```python
from build123d import *

# Parameters (mm, degrees)
SKETCH1_W           = 110
SKETCH1_H           = 50
SKETCH1_R           = 17.5
BOSS_EXTRUDE1_DEPTH = 6
SKETCH2_W           = 110
SKETCH2_H           = 7
BOSS_EXTRUDE2_DEPTH = 65
BOSS_EXTRUDE3_DEPTH = 6
BOSS_EXTRUDE4_DEPTH = 6
CUT_EXTRUDE1_REACH  = 52
SKETCH5_R           = 15
SKETCH6_R           = 3
CUT_EXTRUDE2_DEPTH  = 7
SKETCH7_R           = 2
CUT_EXTRUDE3_DEPTH  = 51


with BuildPart() as part:
    # Sketch1 → Boss-Extrude1 (new body)
    with BuildSketch(Plane(origin=(0, 0, 0), x_dir=(1, 0, 0), z_dir=(0, 1, 0))):
        Rectangle(SKETCH1_W, SKETCH1_H)
        Circle(SKETCH1_R, mode=Mode.SUBTRACT)
    extrude(amount=BOSS_EXTRUDE1_DEPTH)

    # Sketch2 → Boss-Extrude2 (add)
    with BuildSketch(Plane(origin=(0, 6, 0), x_dir=(1, 0, 0), z_dir=(0, 1, 0))):
        with Locations((0, -21.5)):
            Rectangle(SKETCH2_W, SKETCH2_H)
    extrude(amount=BOSS_EXTRUDE2_DEPTH)

    # Sketch3 → Boss-Extrude3 (add)
    with BuildSketch(Plane(origin=(55, 0, 0), x_dir=(0, 0, -1), z_dir=(1, 0, 0))):
        Polygon((-18, 6), (25, 6), (-18, 49), align=None)
    extrude(amount=-BOSS_EXTRUDE3_DEPTH)

    # Sketch4 → Boss-Extrude4 (add)
    with BuildSketch(Plane.ZY.offset(55)):
        Polygon((-25, 6), (18, 6), (18, 49), align=None)
    extrude(amount=-BOSS_EXTRUDE4_DEPTH)

    # Sketch5 → Cut-Extrude1 (cut, up to next)
    with BuildSketch(Plane.XY.offset(25), mode=Mode.PRIVATE) as cut_extrude1_sk1:
        with Locations((0, 46)):
            Circle(SKETCH5_R)
    cut_extrude1_tool1 = extrude(cut_extrude1_sk1.sketch, amount=-CUT_EXTRUDE1_REACH, mode=Mode.PRIVATE) & part.part
    add(cut_extrude1_tool1.solids().sort_by_distance((0, 46, 25))[0], mode=Mode.SUBTRACT)

    # Sketch6 → Cut-Extrude2 (cut, through all)
    with BuildSketch(Plane(origin=(0, 6, 0), x_dir=(1, 0, 0), z_dir=(0, 1, 0))):
        with Locations((-41.329699244, 20)):
            Circle(SKETCH6_R)
        with Locations((-41.329699244, -13)):
            Circle(SKETCH6_R)
        with Locations((41.329699244, -13)):
            Circle(SKETCH6_R)
        with Locations((41.329699244, 20)):
            Circle(SKETCH6_R)
    extrude(amount=-CUT_EXTRUDE2_DEPTH, mode=Mode.SUBTRACT)

    # Sketch7 → Cut-Extrude3 (cut, through all)
    with BuildSketch(Plane.XY.offset(25)):
        with Locations((-27, 65)):
            Circle(SKETCH7_R)
        with Locations((27, 65)):
            Circle(SKETCH7_R)
        with Locations((-27, 11)):
            Circle(SKETCH7_R)
        with Locations((27, 11)):
            Circle(SKETCH7_R)
    extrude(amount=-CUT_EXTRUDE3_DEPTH, mode=Mode.SUBTRACT)


solid = part.part
```
Read the model definition and answer for the solid it produces. Units are mm, in the model's axes. A direction names the side the tool comes from. Coordinates: 2 decimals unless noted, no trailing zeros. Order: outer loops, then holes, each group sorted by start corner. A loop starts at its lowest first (then second) coordinate and runs counter-clockwise, first axis right, second up. Notation, with made-up numbers: (26, 76.25) - (64, 76.25) arc R19 cw to (64, 88.25) - close; hole circle Ø8 at (10, 13). An arc over 180 degrees is marked (long way). Answer as a JSON object with one key per item and string values. Group by question number.
Item 1: The mould has two halves that part along Y. Classify faces 1 (the face through (-13, 0, 16)), 2 (the face through (-25.092, 11.601, 21.549)), 3 (the face through (-49, 18, 6)): +Y half, -Y half, draft (parallel to the pull), parting line (faces both ways), or undercut.
Item 2: Section B-B (y = 46) is taken. Give the vertices of the cut face in (x, z).
Item 3: A tool of negligible diameter and unlimited length cuts with its end or side. For faces 4 (the face through (-13.887, 2.958, 10.648)), 5 (the face through (-0.8, 30.8, 18)), from which of +Z, -Z, +X, -X, +Y, -Y can it reach the whole face along a straight path? Write none if from no direction.
Item 4: Section A-A (x = -27) is taken. Give the vertices of the cut face in (y, z).
Item 5: Section D-D (z = -20) is taken. Give the vertices of the cut face in (x, y), plus the area to 3 significant figures.
Item 6: Flat-ended cylindrical pins translate along their axes: P1, Ø3.5, axis at x = -41.33, z = 13, coming from the -Y side; P2, Ø5, axis at x = 18, y = 19.5, coming from the -Z side; P3, Ø8, axis at x = 41.33, z = -20, coming from the +Y side. Find the tip coordinate at first contact, or state that the pin passes through.
Item 7: Section C-C (z = 0) is taken. Give the vertices of the cut face in (x, y).
Item 8: Consider probe 1 along X at (y, z) = (13.5, -13.5); probe 2 along Y at (x, z) = (-27, 22); probe 3 along Z at (x, y) = (0, 2). Determine where each line is inside the solid, lowest interval first. Write a range as from..to.
Results are:
{
 "1": {"face 1": "-Y half", "face 2": "undercut", "face 3": "draft"},
 "2": {"outline": "(-55, 15) - (-49, 15) - (-49, 18) - (-15, 18) - (-15, 25) - (-55, 25) - close; (15, 18) - (49, 18) - (49, 15) - (55, 15) - (55, 25) - (15, 25) - close"},
 "3": {"face 4": "+Y, -Y", "face 5": "-Z, +Y"},
 "4": {"outline": "(0, -25) - (6, -25) - (6, 18) - (9, 18) - (9, 25) - (0, 25) - close; (13, 18) - (63, 18) - (63, 25) - (13, 25) - close; (67, 18) - (71, 18) - (71, 25) - (67, 25) - close"},
 "5": {"outline": "(-55, 0) - (-44.33, 0) - (-44.33, 6) - (-49, 6) - (-49, 11) - (-55, 11) - close; (-38.33, 0) - (38.33, 0) - (38.33, 6) - (-38.33, 6) - close; (44.33, 0) - (55, 0) - (55, 11) - (49, 11) - (49, 6) - (44.33, 6) - close", "area": "648 mm^2"},
 "6": {"P1": "passes through", "P2": "stops at z = 18", "P3": "stops at y = 6"},
 "7": {"outline": "(-55, 0) - (-17.5, 0) - (-17.5, 6) - (-49, 6) - (-49, 31) - (-55, 31) - close; (17.5, 0) - (55, 0) - (55, 31) - (49, 31) - (49, 6) - (17.5, 6) - close"},
 "8": {"probe 1": "x = -55..-49, 49..55", "probe 2": "y = 0..9, 13..63, 67..71", "probe 3": "z = -25..-17.5, 17.5..25"}
}
